Here's how the part is built. I have some questions about the finished solid (model axes, mm). A direction names the side the tool comes from. Round coordinates to 2 decimals unless told otherwise and drop trailing zeros. Write each loop counter-clockwise with the first axis right and the second up, starting at its lowest first coordinate (ties: lowest second). Pieces come first, ordered by that corner, then holes. Notation, with made-up numbers: M 29,-22.75 L 36,-22.75 A21 cw 36,-13.75 Z; hole C 60.5,4.25 d6. An arc over 180 degrees is marked long. Write item = value, one per line. Start each with the question number.
(1) Will these pins go through, and if not, where does the flat tip stop? pin 1 Ø6 at (x, y) = (7.5, -53.5) entering from +Z; pin 2 Ø1 at (x, z) = (40.5, 34.5) entering from +Y; pin 3 Ø5 at (x, z) = (16.5, 83) entering from -Y.
(2) I want a section at D-D (y = -22). List the corners of the cut face in (x, z) for me, and give its area (3 significant figures).
(3) I want a section at A-A (z = 6.5). List the corners of the cut face in (x, y) for me.
(4) I need wall thicknesses on line 1 along Z through (x, y) = (50, -1.55); line 2 along X through (y, z) = (-3.5, 34.5); line 3 along Y through (x, z) = (9.5, 25.5). Which ranges of each line are inside material? Lowest first, please.
(5) I want a section at C-C (z = 26.5). List the corners of the cut face in (x, y) for me.
(6) I want a section at B-B (x = 46.5). List the corners of the cut face in (y, z) for me.
(7) On a 3-axis mill with a long thin cutter (end or side, diameter ignored), from which of +Z, -Z, +X, -X, +Y, -Y can I reach the whole of each face in a straight line? I mean faces 1 (the flat face through (25, -75, 24)), 2 (the flat face through (28, -8, 84)), 3 (the flat face through (2, -5, 76)), 4 (the flat face through (50, -4.5, 42)), 5 (the flat face through (57, -40, 89)). Say none if no direction works.
(8) If we mould it in two halves opening along Y, with no side actions, what happens to faces 6 (the flat face through (45, -2, 46)), 7 (the flat face through (29, -73, 44)), 8 (the flat face through (25, -5, 59))? For each: released by +Y, released by -Y, zero draft, split by the parting line, or undercut.
```python
from build123d import *

# Parameters (mm, degrees)
SKETCH1_W           = 80
SKETCH1_H           = 60
BOSS_EXTRUDE1_DEPTH = 4
SKETCH3_W           = 5
SKETCH3_H           = 5
BOSS_EXTRUDE2_DEPTH = 85
SKETCH9_W           = 3
SKETCH9_H           = 30
SKETCH9_H_2         = 10
BOSS_EXTRUDE4_DEPTH = 55
FILLET2_R           = 2
SKETCH11_R          = 2
CUT_EXTRUDE2_DEPTH  = 4.5


with BuildPart() as part:
    # Sketch1 → Boss-Extrude1 (new body)
    with BuildSketch(Plane(origin=(0, 0, 0), x_dir=(0, 1, 0), z_dir=(0, 0, 1))):
        with Locations((-40, -30)):
            Rectangle(SKETCH1_W, SKETCH1_H)
    extrude(amount=BOSS_EXTRUDE1_DEPTH)

    # Sketch3 → Boss-Extrude2 (add)
    with BuildSketch(Plane.XY.offset(4)):
        with Locations((2.5, -2.5)):
            Rectangle(SKETCH3_W, SKETCH3_H)
        with Locations((2.5, -77.5)):
            Rectangle(SKETCH3_W, SKETCH3_H)
        Polygon((60, 0), (55, 0), (45, 0), (45, -5), (55, -5), (55, -75), (45, -75), (45, -80), (52.705337411, -80), (60, -80), align=None)
    extrude(amount=BOSS_EXTRUDE2_DEPTH)

    # Sketch9 → Boss-Extrude4 (add)
    with BuildSketch(Plane(origin=(55, 0, 0), x_dir=(0, -1, 0), z_dir=(-1, 0, 0))):
        with Locations((6.5, 24)):
            Rectangle(SKETCH9_W, SKETCH9_H)
        with Locations((6.5, 59)):
            Rectangle(SKETCH9_W, SKETCH9_H)
        with Locations((6.5, 84)):
            Rectangle(SKETCH9_W, SKETCH9_H_2)
        with Locations((73.5, 24)):
            Rectangle(SKETCH9_W, SKETCH9_H)
        with Locations((73.5, 59)):
            Rectangle(SKETCH9_W, SKETCH9_H)
        with Locations((73.5, 84)):
            Rectangle(SKETCH9_W, SKETCH9_H_2)
    extrude(amount=BOSS_EXTRUDE4_DEPTH)

    # Fillet2
    fillet2_edges = [part.edges().sort_by_distance(p)[0] for p in [
        (0, -6.5, 79),
        (0, -73.5, 39),
        (0, -73.5, 9),
        (0, -73.5, 74),
        (0, -73.5, 44),
        (0, -73.5, 79),
        (0, -6.5, 9),
        (0, -6.5, 39),
        (0, -6.5, 44),
        (0, -6.5, 74),
    ]]
    fillet(fillet2_edges, radius=FILLET2_R)

    # Sketch11 → Cut-Extrude2 (cut)
    with BuildSketch(Plane(origin=(0, 0, 0), x_dir=(-1, 0, 0), z_dir=(0, 1, 0))):
        with Locations((-50, 76.5)):
            Circle(SKETCH11_R)
        with Locations((-50, 41.5)):
            Circle(SKETCH11_R)
        with Locations((-50, 6.5)):
            Circle(SKETCH11_R)
    extrude(amount=-CUT_EXTRUDE2_DEPTH, mode=Mode.SUBTRACT)


solid = part.part
```
Returned:
q1.pin_1 = 4
q1.pin_2 = -5
q1.pin_3 = -75
q2.outline = M 0,0 L 60,0 L 60,89 L 55,89 L 55,4 L 0,4 Z
q2.area = 665 mm²
q3.outline = M 0,-80 L 5,-80 L 5,-75 L 0,-75 Z; M 0,-5 L 5,-5 L 5,0 L 0,0 Z; M 45,-80 L 60,-80 L 60,0 L 52,0 L 52,-4.5 L 48,-4.5 L 48,0 L 45,0 L 45,-5 L 55,-5 L 55,-75 L 45,-75 Z
q4.line_1 = 0 to 4.5, 8.5 to 39.5, 43.5 to 74.5, 78.5 to 89
q4.line_2 = 0 to 5, 45 to 60
q4.line_3 = -75 to -72, -8 to -5
q5.outline = M 0,-80 L 5,-80 L 5,-75 L 45,-75 L 45,-80 L 60,-80 L 60,0 L 45,0 L 45,-5 L 5,-5 L 5,0 L 0,0 L 0,-8 L 55,-8 L 55,-72 L 0,-72 Z
q6.outline = M -80,0 L 0,0 L 0,89 L -8,89 L -8,79 L -5,79 L -5,74 L -8,74 L -8,44 L -5,44 L -5,39 L -8,39 L -8,9 L -5,9 L -5,4 L -75,4 L -75,9 L -72,9 L -72,39 L -75,39 L -75,44 L -72,44 L -72,74 L -75,74 L -75,79 L -72,79 L -72,89 L -80,89 Z
q7.face_1 = +Z, -Y
q7.face_2 = +Z, -X
q7.face_3 = -X
q7.face_4 = +Y
q7.face_5 = +Z, +X, -X, +Y, -Y
q8.face_6 = zero draft
q8.face_7 = undercut
q8.face_8 = released by +Y
